Work out the finished part from the listing and answer in its coordinate system (mm). A direction names the side the tool comes from. Round coordinates to 2 decimals unless told otherwise and drop trailing zeros. Order: outer loops, then holes, each group sorted by start corner. A loop starts at its lowest first (then second) coordinate and runs counter-clockwise, first axis right, second up. Notation, with made-up numbers: (64.5, 18.25) - (80.5, 18.25) arc R18 ccw to (80.5, 41.25) - close; hole circle Ø4 at (21, 16.5). An arc over 180 degrees is marked (long way). Answer in a Markdown table with one row per item.
from build123d import *

# Parameters (mm, degrees)
ESQUISSE1_R        = 17
ESQUISSE1_R_2      = 14
ESQUISSE3_W        = 65
ESQUISSE3_H        = 45
ESQUISSE3_R        = 14
ESQUISSE3_R_2      = 2
BOSS_EXTRU_1_DEPTH = 3


with BuildPart() as part:
    # Balayage1: sweep along a path in Esquisse2
    with BuildLine(Plane(origin=(0, 0, 0), x_dir=(0, 0, -1), z_dir=(1, 0, 0))) as balayage1_path:
        ThreePointArc((0, 0), (41.597979746, -15.573593129), (60, -56))
    # Esquisse1 → Balayage1 (sweep)
    with BuildSketch(Plane.XY):
        Circle(ESQUISSE1_R)
        Circle(ESQUISSE1_R_2, mode=Mode.SUBTRACT)
    sweep(path=balayage1_path.line)

    # Esquisse3 → Boss.-Extru.1 (add)
    with BuildSketch(Plane.XY):
        Rectangle(ESQUISSE3_W, ESQUISSE3_H)
        Circle(ESQUISSE3_R, mode=Mode.SUBTRACT)
        with Locations((-23.25, 11.25)):
            Circle(ESQUISSE3_R_2, mode=Mode.SUBTRACT)
        with Locations((-23.25, -11.25)):
            Circle(ESQUISSE3_R_2, mode=Mode.SUBTRACT)
        with Locations((23.25, -11.25)):
            Circle(ESQUISSE3_R_2, mode=Mode.SUBTRACT)
        with Locations((23.25, 11.25)):
            Circle(ESQUISSE3_R_2, mode=Mode.SUBTRACT)
    extrude(amount=BOSS_EXTRU_1_DEPTH)


solid = part.part
1) Find section A-A, the plane x = 23.25. Give the vertices of the cut face in (y, z).
Filled in:
| item | result |
|---|---|
| outline | (-22.5, 0) - (-13.25, 0) - (-13.25, 3) - (-22.5, 3) - close; (-9.25, 0) - (9.25, 0) - (9.25, 3) - (-9.25, 3) - close; (13.25, 0) - (22.5, 0) - (22.5, 3) - (13.25, 3) - close |
2) Which of the six approach directions +Z, -Z, +X, -X, +Y, -Y give full straight-line access (tool end or side, diameter ignored) to faces 4 (the face through (14, 10, 0)), 5 (the face through (12.932, -5.362, 1.479)), 6 (the face through (-32.5, 0, 1))?
Filled in:
| item | result |
|---|---|
| face 4 | none |
| face 5 | +Z |
| face 6 | +Z, -Z, -X, +Y, -Y |
3) Find section B-B, the plane y = -11.25. Give the number of separate pieces and of enclosed holes in the cut face, then the cut area to 3 significant figures.
Filled in:
| item | result |
|---|---|
| separate pieces | 3 |
| enclosed holes | 0 |
| area | 593 mm^2 |
4) Find section C-C, the plane x = -28. Give the vertices of the cut face in (y, z).
Filled in:
| item | result |
|---|---|
| outline | (-22.5, 0) - (22.5, 0) - (22.5, 3) - (-22.5, 3) - close |
5) Find the intervals of material crossed by probe 1 along X at (y, z) = (11, 1); probe 2 along X at (y, z) = (-9, -33.5); probe 3 along Y at (x, z) = (0, 1.25), in increasing order. Write a range as from..to.
Filled in:
| item | result |
|---|---|
| probe 1 | x = -32.5..-25.23, -21.27..-8.66, 8.66..21.27, 25.23..32.5 |
| probe 2 | x = -17..-14, 14..17 |
| probe 3 | y = -22.5..-14, 14..22.5 |
6) Each of these flat-tipped pins is pushed along its axis until it touches: pin 1 (4 mm diameter, centred on x = 3, z = -12.5, fed in from -Y); pin 2 (3.5 mm diameter, centred on x = -1.5, z = 2, fed in from -Y); pin 3 (5 mm diameter, centred on x = 23.25, y = 11.25, fed in from -Z). Where does it stop, or does it pass through?
Filled in:
| item | result |
|---|---|
| pin 1 | stops at y = -18.7 |
| pin 2 | stops at y = -22.5 |
| pin 3 | stops at z = 0 |
7) The mould has two halves that part along Y. Classify faces 1 (the face through (0, -22.5, 1)), 2 (the face through (0, 22.5, 1)), 3 (the face through (-24.724, 12.602, 1.479)): released by +Y, released by -Y, zero draft, split by the parting line, or undercut.
Filled in:
| item | result |
|---|---|
| face 1 | released by -Y |
| face 2 | released by +Y |
| face 3 | undercut |
